Read the model definition and answer for the solid it produces. Units are mm, in the model's axes. Face numbers are marked on the shaded views. A direction names the side the tool comes from. Round coordinates to 2 decimals unless told otherwise and drop trailing zeros. Write each loop counter-clockwise with the first axis right and the second up, starting at its lowest first coordinate (ties: lowest second). Pieces come first, ordered by that corner, then holes. Notation, with made-up numbers: (41, -27.75) -> (97, -27.75) arc R23 cw to (97, -2.75) -> close; hole circle Ø3 at (61.25, 57). An arc over 180 degrees is marked (long way). Return JSON: item names as keys, results as strings.
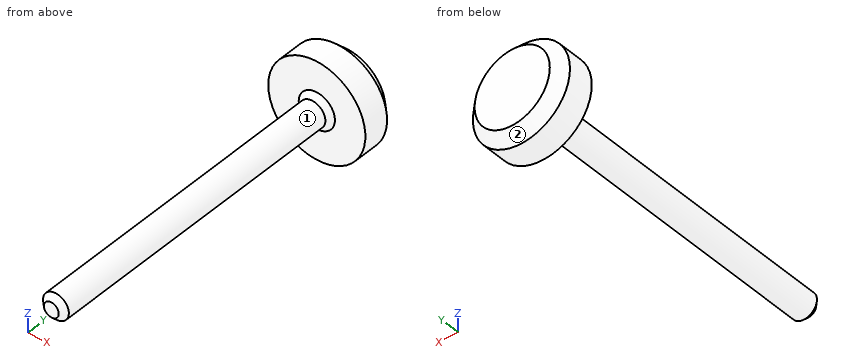
from build123d import *

# Parameters (mm, degrees)
CHAMFER3_SIZE = 1


with BuildPart() as part:
    # Sketch2 → Revolve1 (revolve)
    with BuildSketch(Plane.XY):
        Polygon((0, 22.313788144), (-7.264862559, 22.313788144), (-9.386182903, 20.192467801), (-9.386182903, 15.192467801), (-2.5, 15.192467801), (-2.5, -44.807532199), (-1.439339828, -45.868192371), (0, -45.868192371), align=None)
    revolve(axis=Axis((0, 22.313788144, 0), (0, -1, 0)))

    # Chamfer3
    chamfer3_edges = [part.edges().sort_by_distance(p)[0] for p in [
        (2.5, 15.192467801, 0),
    ]]
    chamfer(chamfer3_edges, length=CHAMFER3_SIZE)


solid = part.part
Item 1: Section D-D (y = 17) is taken. Give the vertices of the cut face in (x, z), then the cut area to 3 significant figures.
Worked answers:
{"outline": "circle Ø18.77 at (0, 0)", "area": "277 mm2"}
Item 2: Flat-ended cylindrical pins translate along their axes: pin 1 (1.5 mm diameter, centred on y = 14, z = 2, fed in from +X); pin 2 (1.5 mm diameter, centred on x = -2, y = 2.5, fed in from -Z); pin 3 (4 mm diameter, centred on x = -2, y = -2, fed in from -Z). Find the tip coordinate at first contact, or state that the pin passes through.
Worked answers:
{"pin 1": "stops at x = 2.47", "pin 2": "stops at z = -2.17", "pin 3": "stops at z = -2.5"}
Item 3: Section C-C (y = -30.5) is taken. Give the vertices of the cut face in (x, z), then the cut area to 3 significant figures.
Worked answers:
{"outline": "circle Ø5 at (0, 0)", "area": "19.6 mm2"}
Item 4: Section B-B (z = 0) is taken. Give the vertices of the cut face in (x, y).
Worked answers:
{"outline": "(-9.39, 15.19) -> (-3.5, 15.19) -> (-2.5, 14.19) -> (-2.5, -44.81) -> (-1.44, -45.87) -> (1.44, -45.87) -> (2.5, -44.81) -> (2.5, 14.19) -> (3.5, 15.19) -> (9.39, 15.19) -> (9.39, 20.19) -> (7.26, 22.31) -> (-7.26, 22.31) -> (-9.39, 20.19) -> close"}
Item 5: A tool of negligible diameter and unlimited length cuts with its end or side. For the marked faces 1 and 2, from which of +Z, -Z, +X, -X, +Y, -Y can it reach the whole face along a straight path? Write none if from no direction.
Worked answers:
{"face 1": "-Y", "face 2": "+Y"}
Item 6: Section A-A (x = 0) is taken. Give the vertices of the cut face in (y, z), then the cut area to 3 significant figures.
Worked answers:
{"outline": "(-45.87, -1.44) -> (-44.81, -2.5) -> (14.19, -2.5) -> (15.19, -3.5) -> (15.19, -9.39) -> (20.19, -9.39) -> (22.31, -7.26) -> (22.31, 7.26) -> (20.19, 9.39) -> (15.19, 9.39) -> (15.19, 3.5) -> (14.19, 2.5) -> (-44.81, 2.5) -> (-45.87, 1.44) -> close", "area": "434 mm2"}
Item 7: Straight lines are drawn through the part: L1, parallel to X at y = 3.5, z = 0.25; L2, parallel to Y at x = -4.25, z = -1.75; L3, parallel to Z at x = -1.75, y = -40. For each, find the intervals that lie inside material, in ascending order. Write a range as [from, to].
Worked answers:
{"L1": "x = [-2.49, 2.49]", "L2": "y = [15.19, 22.31]", "L3": "z = [-1.79, 1.79]"}
